from build123d import *

# Parameters (mm, degrees)
F0_R            = 11
F1_DEPTH        = 7
F1_COPIES_COUNT = 3


# Not quite as in the source:
# - a pattern or mirror of a feature is missing from the dataset's text; its kind, count and spacing are read off the source's solid


with BuildPart() as f1:
    # F0 (on Top) → F1 (new body)
    with BuildSketch(Plane.XY):
        with BuildLine():
            ThreePointArc((0, 11), (7.7781745931, 7.7781745931), (11, 0))
            ThreePointArc((11, 0), (7.7781745931, -7.7781745931), (0, -11))
            Line((0, -11), (0, -18.5))
            Line((0, -18.5), (40, -18.5))
            ThreePointArc((40, -18.5), (58.5, 0), (40, 18.5))
            Line((40, 18.5), (0, 18.5))
            Line((0, 18.5), (0, 11))
        make_face()
        with Locations((40, 0)):
            Circle(F0_R, mode=Mode.SUBTRACT)
    extrude(amount=F1_DEPTH)

    # F1_copies: F1 ×3 about axis
    f1_copies_axis = Axis((0, 0, 0), (0, 0, 1))


with BuildPart() as f1_1:
    add(f1.part)
    for i in range(1, F1_COPIES_COUNT):
        add(f1.part.rotate(f1_copies_axis, i * 360 / F1_COPIES_COUNT))


solid = f1_1.part
Input: part model. Units: mm. Frame: model coordinates. A direction names the side the tool comes from. Give positions to 0.01 mm unless a question says otherwise; leave off trailing zeros. Loops run counter-clockwise (first coordinate to the right, second up) from the corner with the lowest first, then second, coordinate; pieces in that order, holes last. Notation, with made-up numbers: M -23.5,48 L 29.5,48 A28 ccw 29.5,72 Z; hole C 28,60.5 d9. An arc over 180 degrees is marked long. Use one line per item in the form item = value.
1. Line query: L1, parallel to Y at x = 40, z = 4; L2, parallel to X at y = -1, z = 3; L3, parallel to X at y = 7, z = 2.5. Output: solid intervals per line, ascending.
Numbers:
L1 = -18.5 to -11, 11 to 18.5
L2 = -21.94 to -10.95, 10.95 to 29.05, 50.95 to 58.47
L3 = -25.4 to -8.49, 8.49 to 31.51, 48.49 to 57.12
2. Reachability of faces 1 (the face through (26, 18.5, 3)), 2 (the face through (58.496, -0.407, 3.451)), 3 (the face through (-28.59, -12.52, 3.45)) from +Z, -Z, +X, -X, +Y, -Y: full face, straight path, thin tool, end or side. Return the list, or none.
Numbers:
face_1 = +Z, -Z, +X, +Y
face_2 = +Z, -Z, +X
face_3 = +Z, -Z, -X
3. First-contact query: pin 1 (1 mm diameter, centred on x = -10, z = 1, fed in from -Y); pin 2 (1 mm diameter, centred on y = 40, z = 4, fed in from -X); pin 3 (20 mm diameter, centred on x = 40, y = 0, fed in from +Z); pin 4 (1 mm diameter, centred on x = 4, z = 4.5, fed in from -Y). Flat tips, straight axial feed; report the tip coordinate or a pass-through.
Numbers:
pin_1 = -50.52
pin_2 = -37.85
pin_3 = through
pin_4 = -30.94
4. Section query C-C, the plane z = 2.25. Return the cut outline in (x, y).
Numbers:
outline = M -36.02,-25.39 A18.5 ccw -3.98,-43.89 L 10.68,-18.5 L 40,-18.5 A18.5 ccw 40,18.5 L 10.68,18.5 L -3.98,43.89 A18.5 ccw -36.02,25.39 L -21.36,0 Z; hole C -20,-34.64 d22; hole C -20,34.64 d22; hole C 0,0 d22; hole C 40,0 d22
5. Section query B-B, the plane y = 42.5. Return the cut outline in (x, z), and give its area (3 significant figures).
Numbers:
outline = M -36.75,0 L -27.7,0 L -27.7,7 L -36.75,7 Z; M -12.3,0 L -3.18,0 L -3.18,7 L -12.3,7 Z
area = 127 mm²
6. Section query A-A, the plane x = -20. Return the cut outline in (y, z), and give its area (3 significant figures).
Numbers:
outline = M -53.14,0 L -45.64,0 L -45.64,7 L -53.14,7 Z; M -23.64,0 L 23.64,0 L 23.64,7 L -23.64,7 Z; M 45.64,0 L 53.14,0 L 53.14,7 L 45.64,7 Z
area = 436 mm²
7. Pull-direction query (X, two-part tool) for faces 4 (the face through (-29.6, -50.455, 3.451)), 5 (the face through (50.161, -4.213, 3.451)), 6 (the face through (25, -18.5, 3)), 7 (the face through (-28.794, 12.873, 3.451)); classes: released by +X, released by -X, zero draft, split by the parting line, or undercut.
Numbers:
face_4 = split by the parting line
face_5 = undercut
face_6 = zero draft
face_7 = released by -X
8. Section query D-D, the plane x = 3.5. Return the cut outline in (y, z).
Numbers:
outline = M -30.94,0 L -10.43,0 L -10.43,7 L -30.94,7 Z; M 10.43,0 L 30.94,0 L 30.94,7 L 10.43,7 Z
